```python
from build123d import *

# Parameters (mm, degrees)
F0_R     = 8.001
F0_R_2   = 5.08
F1_DEPTH = 152.4
F2_R     = 8.001
F2_R_2   = 5.08
F3_ANGLE = 45
F4_R     = 8.001
F4_R_2   = 5.08
F5_DEPTH = 19.05
F6_R     = 8.001
F6_R_2   = 5.08
F7_ANGLE = 45
F8_R     = 8.001
F8_R_2   = 5.08
F9_DEPTH = 38.1


with BuildPart() as f1:
    # F0 (on Front) → F1 (new body)
    with BuildSketch(Plane.XZ):
        Circle(F0_R)
        Circle(F0_R_2, mode=Mode.SUBTRACT)
    extrude(amount=F1_DEPTH)

    # F2 (on face) → F3 (revolve)
    with BuildSketch(Plane.XZ.offset(152.4)):
        Circle(F2_R)
        Circle(F2_R_2, mode=Mode.SUBTRACT)
    revolve(axis=Axis((1.8257172778, -152.4, -19.05), (1, 0, 0)), revolution_arc=F3_ANGLE)

    # F4 (on face) → F5 (join)
    with BuildSketch(Plane(origin=(0, -85.725, -85.725), x_dir=(1, 0, 0), z_dir=(0, -0.7071067812, -0.7071067812))):
        with Locations((0, 113.3426892712)):
            Circle(F4_R)
        with Locations((0, 113.3426892712)):
            Circle(F4_R_2, mode=Mode.SUBTRACT)
    extrude(amount=F5_DEPTH)

    # F6 (on face) → F7 (revolve)
    with BuildSketch(Plane(origin=(0, -99.1953841816, -99.1953841816), x_dir=(1, 0, 0), z_dir=(0, -0.7071067812, -0.7071067812))):
        with Locations((0, 113.3426892712)):
            Circle(F6_R)
        with Locations((0, 113.3426892712)):
            Circle(F6_R_2, mode=Mode.SUBTRACT)
    revolve(axis=Axis((0.5769948475, -192.8111525448, -5.5796158184), (-1, 0, 0)), revolution_arc=F7_ANGLE)

    # F8 (on face) → F9 (join)
    with BuildSketch(Plane.XZ.offset(192.8111525448)):
        with Locations((0, -24.6296158184)):
            Circle(F8_R)
        with Locations((0, -24.6296158184)):
            Circle(F8_R_2, mode=Mode.SUBTRACT)
    extrude(amount=F9_DEPTH)


solid = f1.part
```
Read the model definition and answer for the solid it produces. Units are mm, in the model's axes. A direction names the side the tool comes from. Give positions to 0.01 mm unless a question says otherwise; leave off trailing zeros. Loops run counter-clockwise (first coordinate to the right, second up) from the corner with the lowest first, then second, coordinate; pieces in that order, holes last.
Item 1: For faces 1 (the cylindrical face through (-0.661, -75.133, 5.037)), 2 (the flat face through (5, 0, -2)), 3 (the cylindrical face through (-1.042, -211.594, -16.697)), determine the directions among +Z, -Z, +X, -X, +Y, -Y from which every point of the face is accessible in a straight line to the end or side of a thin tool.
Item 2: The part is cut by section B-B (y = -75). Write down the section's boundary in (x, z), and give its area (3 significant figures).
Item 3: The part is cut by section A-A (x = 0). Write down the section's boundary in (y, z).
Item 4: Find the intervals of material crossed by line 1 along Z through (x, y) = (0, -86); line 2 along Z through (x, y) = (0, -216); line 3 along X through (y, z) = (-97, -3.5), in increasing order.
Item 5: The mould has two halves that part along Z. Classify faces 4 (the cylindrical face through (-1.04, -178.12, -6.61)), 5 (the cylindrical face through (-1.1, -211.59, -29.59)), 6 (the flat face through (0, -230.911, -30)), 7 (the cylindrical face through (-1.101, -169.005, -15.727)): released by +Z, released by -Z, zero draft, split by the parting line, or undercut.
Item 6: Each of these flat-tipped pins is pushed along its axis until it touches: pin 1 Ø4 at (x, y) = (2.5, -50) entering from +Z; pin 2 Ø2 at (x, y) = (6, -94.5) entering from -Z; pin 3 Ø6 at (x, z) = (-6.5, -16.5) entering from +Y. Where does it stop, or does it pass through?
Taken from the geometry:
1. face 1: +Y
1. face 2: +Z, -Z, +X, -X, +Y
1. face 3: -Y
2. outline: circle Ø16 at (0, 0); hole circle Ø10.16 at (0, 0)
2. area: 120 mm2
3. outline: (-230.91, -32.63) - (-192.81, -32.63) arc R27.05 ccw to (-173.68, -24.71) - (-160.21, -11.24) arc R11.05 cw to (-152.4, -8) - (0, -8) - (0, -5.08) - (-152.4, -5.08) arc R13.97 ccw to (-162.28, -9.17) - (-175.75, -22.64) arc R24.13 cw to (-192.81, -29.71) - (-230.91, -29.71) - close; (-230.91, -19.55) - (-192.81, -19.55) arc R13.97 ccw to (-182.93, -15.46) - (-169.46, -1.99) arc R24.13 cw to (-152.4, 5.08) - (0, 5.08) - (0, 8) - (-152.4, 8) arc R27.05 ccw to (-171.53, 0.08) - (-185, -13.39) arc R11.05 cw to (-192.81, -16.63) - (-230.91, -16.63) - close
4. line 1: z = -8 to -5.08, 5.08 to 8
4. line 2: z = -32.63 to -29.71, -19.55 to -16.63
4. line 3: x = -7.19 to -3.68, 3.68 to 7.19
5. face 4: split by the parting line
5. face 5: undercut
5. face 6: zero draft
5. face 7: undercut
6. pin 1: stops at z = 7.99
6. pin 2: stops at z = -6.25
6. pin 3: stops at y = -165.2
